CAD build for the part. Positions are in the model's coordinates, mm. A direction names the side the tool comes from. Round coordinates to 2 decimals unless told otherwise and drop trailing zeros. Order: outer loops, then holes, each group sorted by start corner. A loop starts at its lowest first (then second) coordinate and runs counter-clockwise, first axis right, second up. Notation, with made-up numbers: M 5,-4 L 9,-4 A19 cw 9,31 Z; hole C 49.25,-29.5 d5. An arc over 180 degrees is marked long. Answer as a JSON object with one key per item and string values. Group by question number.
```python
from build123d import *

# Parameters (mm, degrees)
SKETCH_1_R                     = 54
FLOOR_D108_T3_DEPTH            = 3
SKETCH_2_R                     = 54
SKETCH_2_R_2                   = 51
RIM_OD108_ID102_H24_DEPTH      = 24
SKETCH_3_R                     = 4.5
SENSOR_FIXED_POSTS_DEPTH       = 14
SKETCH_4_R                     = 2.15
M4_FIXED_MOUNT_CLEARANCE_DEPTH = 14


with BuildPart() as part:
    # 草图1 → Floor_D108_T3 (new body)
    with BuildSketch(Plane(origin=(0, 0, 0), x_dir=(1, 0, 0), z_dir=(0, 1, 0))):
        with Locations(Location((0, 0, 0), (0, 0, 270))):
            Circle(SKETCH_1_R)
    extrude(amount=FLOOR_D108_T3_DEPTH)

    # 草图2 → Rim_OD108_ID102_H24 (add)
    with BuildSketch(Plane(origin=(0, 0, 0), x_dir=(1, 0, 0), z_dir=(0, 1, 0))):
        with Locations(Location((0, 0, 0), (0, 0, 270))):
            Circle(SKETCH_2_R)
        with Locations(Location((0, 0, 0), (0, 0, 270))):
            Circle(SKETCH_2_R_2, mode=Mode.SUBTRACT)
    extrude(amount=RIM_OD108_ID102_H24_DEPTH)

    # 草图3 → Sensor_fixed_posts (add)
    with BuildSketch(Plane(origin=(0, 0, 0), x_dir=(1, 0, 0), z_dir=(0, 1, 0))):
        with Locations(Location((22, 0, 0), (0, 0, 270))):
            Circle(SKETCH_3_R)
        with Locations(Location((32, 0, 0), (0, 0, 270))):
            Circle(SKETCH_3_R)
    extrude(amount=SENSOR_FIXED_POSTS_DEPTH)

    # 草图4 → M4_fixed_mount_clearance (cut)
    with BuildSketch(Plane(origin=(0, 0, 0), x_dir=(1, 0, 0), z_dir=(0, 1, 0))):
        with Locations(Location((22, 0, 0), (0, 0, 270))):
            Circle(SKETCH_4_R)
        with Locations(Location((32, 0, 0), (0, 0, 270))):
            Circle(SKETCH_4_R)
    extrude(amount=M4_FIXED_MOUNT_CLEARANCE_DEPTH, mode=Mode.SUBTRACT)


solid = part.part
```
Item 1: Drill centre lines: line 1 (X direction, y = 4.75, z = 0); line 2 (X direction, y = 17.75, z = 0); line 3 (Y direction, x = -41.5, z = -23). Where is each one in solid material? Low to high. Write a range as [from, to].
Item 2: Two-plate mould, pull along X, no slides. Class faces 3 (the face through (-52.716, 11.832, -11.706)), 4 (the face through (27.61, 8.42, -0.98)), 5 (the face through (1, 0, -1)): +X half, -X half, draft (parallel to the pull), parting line (faces both ways), or undercut.
Item 3: 3-axis set-ups, long thin cutter, end or side, ignore diameter. For faces 1 (the face through (1, 3, -1)), 2 (the face through (19.9, 6.9, -0.47)): which of +Z, -Z, +X, -X, +Y, -Y reach the whole face in a straight line?
Item 4: Cut at C-C, the plane y = 19. Give the cut face in (x, z), and give its area (3 significant figures).
Item 5: Cut at B-B, the plane x = 22. Give the cut face in (y, z), and give its area (3 significant figures).
Item 6: Flat gauge pins, fed straight in: pin 1 Ø6 at (x, z) = (-1.5, -39.5) entering from +Y; pin 2 Ø7 at (x, z) = (32.5, -2) entering from +Y; pin 3 Ø3 at (x, y) = (-4.5, 10) entering from -Z. Where does each tip first touch, or does it go through?
Item 7: Cut at A-A, the plane z = 0. Give the cut face in (x, y), and give its area (3 significant figures).
Item 8: Cut at D-D, the plane z = 34. Give the cut face in (x, y), and give its area (3 significant figures).
Response values:
{
 "1": {"line 1": "[-54, -51], [17.5, 19.85], [24.15, 26.5], [27.5, 29.85], [34.15, 36.5], [51, 54]", "line 2": "[-54, -51], [51, 54]", "line 3": "[0, 3]"},
 "2": {"face 3": "parting line", "face 4": "undercut", "face 5": "draft"},
 "3": {"face 1": "+Y", "face 2": "+Y, -Y"},
 "4": {"outline": "C 0,0 d108; hole C 0,0 d102", "area": "990 mm^2"},
 "5": {"outline": "M 0,-49.32 L 24,-49.32 L 24,-46.01 L 3,-46.01 L 3,-4.5 L 14,-4.5 L 14,-2.15 L 0,-2.15 Z; M 0,2.15 L 14,2.15 L 14,4.5 L 3,4.5 L 3,46.01 L 24,46.01 L 24,49.32 L 0,49.32 Z", "area": "473 mm^2"},
 "6": {"pin 1": "y = 3", "pin 2": "y = 14", "pin 3": "z = -53.92"},
 "7": {"outline": "M -54,0 L 19.85,0 L 19.85,14 L 17.5,14 L 17.5,3 L -51,3 L -51,24 L -54,24 Z; M 24.15,0 L 29.85,0 L 29.85,14 L 27.5,14 L 27.5,3 L 26.5,3 L 26.5,14 L 24.15,14 Z; M 34.15,0 L 54,0 L 54,24 L 51,24 L 51,3 L 36.5,3 L 36.5,14 L 34.15,14 Z", "area": "528 mm^2"},
 "8": {"outline": "M -41.95,0 L 41.95,0 L 41.95,24 L 38.01,24 L 38.01,3 L -38.01,3 L -38.01,24 L -41.95,24 Z", "area": "417 mm^2"}
}
